from build123d import *

# Parameters (mm, degrees)
SKETCH010_W         = 26
SKETCH010_H         = 30
SKETCH010_R         = 1.6
SKETCH010_W_2       = 23
SKETCH010_H_2       = 1
PAD009_DEPTH        = 2
PAD009_FACE3_W      = 26
PAD009_FACE3_H      = 2
PAD010_DEPTH        = 2
PAD010_FACE8_W      = 2
PAD010_FACE8_H      = 26
PAD011_DEPTH        = 18
PAD012_DEPTH        = 26
SKETCH012_R         = 1.6
POCKET006_DEPTH     = 33.561
PAD013_DEPTH        = 1.2
LINEARPATTERN_COUNT = 2
LINEARPATTERN_PITCH = 24.8


with BuildPart() as part:
    # Sketch010 → Pad009 (new body)
    with BuildSketch(Plane.XY):
        Rectangle(SKETCH010_W, SKETCH010_H)
        with Locations((0, 10.4)):
            Circle(SKETCH010_R, mode=Mode.SUBTRACT)
        with Locations((0, -4.6)):
            Circle(SKETCH010_R, mode=Mode.SUBTRACT)
        with Locations((0, -12.5)):
            Rectangle(SKETCH010_W_2, SKETCH010_H_2, mode=Mode.SUBTRACT)
    extrude(amount=PAD009_DEPTH)

    # Pad009 Face3 → Pad010 (add)
    with BuildSketch(Plane(origin=(0, -15, 1), x_dir=(-1, 0, 0), z_dir=(0, -1, 0))):
        Rectangle(PAD009_FACE3_W, PAD009_FACE3_H)
    extrude(amount=PAD010_DEPTH)

    # Pad010 Face8 → Pad011 (add)
    with BuildSketch(Plane(origin=(0, -16, 0), x_dir=(0, -1, 0), z_dir=(0, 0, -1))):
        Rectangle(PAD010_FACE8_W, PAD010_FACE8_H)
    extrude(amount=PAD011_DEPTH)

    # Sketch011 (on Face16 of Pad011) → Pad012 (join)
    with BuildSketch(Plane(origin=(-13, 0, 0), x_dir=(0, -1, 0), z_dir=(-1, 0, 0))):
        Polygon((17, -8), (17, -3.26), (18.56, -5.06), (18.56, -10.94), (17, -12.74), align=None)
    extrude(amount=-PAD012_DEPTH)

    # Sketch012 (on Face25 of Pad012) → Pocket006 (cut, through all)
    with BuildSketch(Plane.XZ.offset(18.56)):
        with Locations((-7, -8)):
            Circle(SKETCH012_R)
        with Locations((7, -8)):
            Circle(SKETCH012_R)
    extrude(amount=-POCKET006_DEPTH, mode=Mode.SUBTRACT)

    # Sketch013 (on Face16 of Pocket006) → Pad013 (join)
    with BuildSketch(Plane(origin=(-13, 0, 0), x_dir=(0, -1, 0), z_dir=(-1, 0, 0))):
        Polygon((-15, 0), (15, -18), (15, 0), align=None)
    pad013 = extrude(amount=-PAD013_DEPTH)

    # LinearPattern: Pad013 ×2
    with Locations(*[(i * LINEARPATTERN_PITCH, 0, 0) for i in range(1, LINEARPATTERN_COUNT)]):
        add(pad013)


with BuildPart() as part_1:
    # Body002 placement: moved
    add(part.part.moved(Location((-25, 78, 0))))


solid = part_1.part
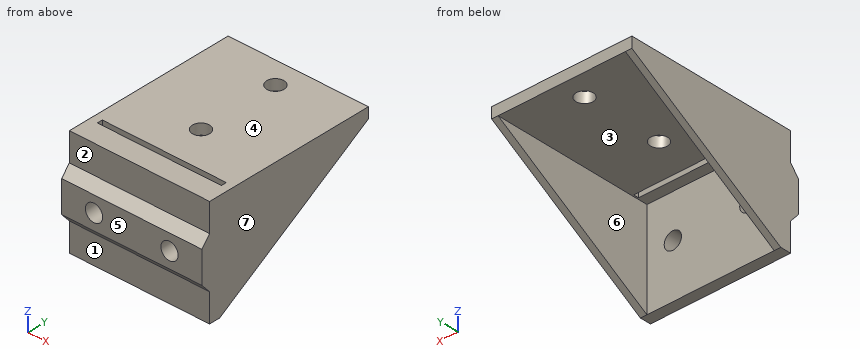
CAD build for the part. Positions are in the model's coordinates, mm. Face numbers are marked on the shaded views. A direction names the side the tool comes from. Round coordinates to 2 decimals unless told otherwise and drop trailing zeros. Write each loop counter-clockwise with the first axis right and the second up, starting at its lowest first coordinate (ties: lowest second). Pieces come first, ordered by that corner, then holes. Notation, with made-up numbers: M -5.75,50.25 L 41.25,50.25 A10 cw 41.25,58.25 Z; hole C 67.25,67.25 d8. An arc over 180 degrees is marked long. Put each result on its own line as item: value. Start each with the question number.
1) Saw through at D-D, the plane z = -8. Write the cut outline in (x, y), and give its area (3 significant figures).
2) 3-axis set-ups, long thin cutter, end or side, ignore diameter. For the marked faces 1, 2, 3 and 4: which of +Z, -Z, +X, -X, +Y, -Y reach the whole face in a straight line?
3) Pin check, flat tips, straight feed: pin 1 Ø1.6 at (x, z) = (-20, 1.5) entering from -Y; pin 2 Ø4 at (x, z) = (-31, -6) entering from +Y; pin 3 Ø12 at (x, y) = (-28.5, 81.5) entering from -Z. Stop position of each tip, or through.
4) Saw through at B-B, the plane x = -22. Write the cut outline in (y, z), and give its area (3 significant figures).
5) Drill centre lines: probe 1 along Y at (x, z) = (-25, 1.1); probe 2 along X at (y, z) = (71, -3.75); probe 3 along Z at (x, y) = (-18, 61.4). Where is each one in solid material? Low to high. Write a range as [from, to].
6) Saw through at C-C, the plane x = -18. Write the cut outline in (y, z).
7) Saw through at A-A, the plane y = 73.4. Write the cut outline in (x, z).
8) Pull direction X, two halves, no side cores. Call the marked faces 5, 6 and 7: pulls with the +X half, pulls with the -X half, needs draft (parallel to the pull), parting line crosses it, or undercut.
Resolved:
1. outline: M -38,59.44 L -33.6,59.44 L -33.6,63 L -36.8,63 L -36.8,79.67 L -38,79.67 Z; M -30.4,59.44 L -19.6,59.44 L -19.6,63 L -30.4,63 Z; M -16.4,59.44 L -12,59.44 L -12,79.67 L -13.2,79.67 L -13.2,63 L -16.4,63 Z
1. area: 110 mm²
2. face 1: -Z, +X, -X, -Y
2. face 2: +Z, +X, -X, -Y
2. face 3: -Z, +Y
2. face 4: +Z, +X, -X, +Y, -Y
3. pin 1: y = 61
3. pin 2: y = 63
3. pin 3: z = 0
4. outline: M 59.44,-10.94 L 61,-12.74 L 61,-18 L 63,-18 L 63,0 L 65,0 L 65,2 L 61,2 L 61,-3.26 L 59.44,-5.06 Z; M 66,0 L 93,0 L 93,2 L 66,2 Z
4. area: 110 mm²
5. probe 1: [61, 65], [66, 71.8], [75, 86.8], [90, 93]
5. probe 2: [-38, -36.8], [-13.2, -12]
5. probe 3: [-18, -9.6], [-6.4, 2]
6. outline: M 59.44,-10.94 L 61,-12.74 L 61,-18 L 63,-18 L 63,-9.6 L 59.44,-9.6 Z; M 59.44,-6.4 L 63,-6.4 L 63,0 L 65,0 L 65,2 L 61,2 L 61,-3.26 L 59.44,-5.06 Z; M 66,0 L 93,0 L 93,2 L 66,2 Z
7. outline: M -38,-11.76 L -36.8,-11.76 L -36.8,0 L -26.6,0 L -26.6,2 L -38,2 Z; M -23.4,0 L -13.2,0 L -13.2,-11.76 L -12,-11.76 L -12,2 L -23.4,2 Z
8. face 5: needs draft
8. face 6: undercut
8. face 7: pulls with the +X half
